Input: part model. Units: mm. Frame: model coordinates. Round coordinates to 2 decimals unless told otherwise and drop trailing zeros. Loops run counter-clockwise (first coordinate to the right, second up) from the corner with the lowest first, then second, coordinate; pieces in that order, holes last. Notation, with made-up numbers: (18, 68.5) -> (35, 68.5) arc R20 ccw to (35, 89.5) -> close; hole circle Ø4 at (58, 14). An arc over 180 degrees is marked (long way). Answer as a JSON object with one key per item and string values.
```python
from build123d import *


with BuildPart() as part:
    # Sketch → Revolution (revolve)
    with BuildSketch(Plane.YZ):
        with BuildLine():
            ThreePointArc((-5.4, 23.5), (-5.824264, 23.324264), (-6, 22.9))
            Line((-6, 13.1), (-6, 22.9))
            ThreePointArc((-6, 13.1), (-5.824264, 12.675736), (-5.4, 12.5))
            Line((5.4, 12.5), (-5.4, 12.5))
            ThreePointArc((5.4, 12.5), (5.824264, 12.675736), (6, 13.1))
            Line((6, 22.9), (6, 13.1))
            ThreePointArc((6, 22.9), (5.824264, 23.324264), (5.4, 23.5))
            Line((-5.4, 23.5), (5.4, 23.5))
        make_face()
    revolve(axis=Axis((0, 0, 0), (0, 1, 0)))


solid = part.part
```
1) Ray query, probe 1 along X at (y, z) = (3, 0); probe 2 along Z at (x, y) = (-5, 1); probe 3 along X at (y, z) = (4.5, 6.5). Return the intervals inside material, ascending.
Output:
{"probe 1": "x = -23.5 to -12.5, 12.5 to 23.5", "probe 2": "z = -22.96 to -11.46, 11.46 to 22.96", "probe 3": "x = -22.58 to -10.68, 10.68 to 22.58"}
2) Draft query along Z for faces 1 (the face through (-10, 6, 10)), 2 (the face through (7.1, 0.1, 22.4)), 3 (the face through (3.755, -0.076, 11.923)). Return one class per face: +Z half, -Z half, draft (parallel to the pull), parting line (faces both ways), or undercut.
Output:
{"face 1": "draft", "face 2": "parting line", "face 3": "undercut"}
3) Section A-A, the plane x = 0. Output: boundary loops of the cut face in (y, z).
Output:
{"outline": "(-6, -22.9) arc R0.6 ccw to (-5.4, -23.5) -> (5.4, -23.5) arc R0.6 ccw to (6, -22.9) -> (6, -13.1) arc R0.6 ccw to (5.4, -12.5) -> (-5.4, -12.5) arc R0.6 ccw to (-6, -13.1) -> close; (-6, 13.1) arc R0.6 ccw to (-5.4, 12.5) -> (5.4, 12.5) arc R0.6 ccw to (6, 13.1) -> (6, 22.9) arc R0.6 ccw to (5.4, 23.5) -> (-5.4, 23.5) arc R0.6 ccw to (-6, 22.9) -> close"}
4) Section B-B, the plane z = 0. Output: boundary loops of the cut face in (x, y).
Output:
{"outline": "(-23.5, -5.4) arc R0.6 ccw to (-22.9, -6) -> (-13.1, -6) arc R0.6 ccw to (-12.5, -5.4) -> (-12.5, 5.4) arc R0.6 ccw to (-13.1, 6) -> (-22.9, 6) arc R0.6 ccw to (-23.5, 5.4) -> close; (12.5, -5.4) arc R0.6 ccw to (13.1, -6) -> (22.9, -6) arc R0.6 ccw to (23.5, -5.4) -> (23.5, 5.4) arc R0.6 ccw to (22.9, 6) -> (13.1, 6) arc R0.6 ccw to (12.5, 5.4) -> close"}
5) Section C-C, the plane y = -0.25. Output: boundary loops of the cut face in (x, z).
Output:
{"outline": "circle Ø47 at (0, 0); hole circle Ø25 at (0, 0)"}
6) Contact query for flat-ended pins moving along their axis: P1, Ø2, axis at y = 3, z = 16.5, coming from the +X side; P2, Ø3, axis at y = -3.5, z = -12, coming from the -X side; P3, Ø2, axis at x = 13.5, y = 1.5, coming from the -Z side. Output: stop coordinate, or through.
Output:
{"P1": "stops at x = 17.66", "P2": "stops at x = -21.02", "P3": "stops at z = -19.9"}
